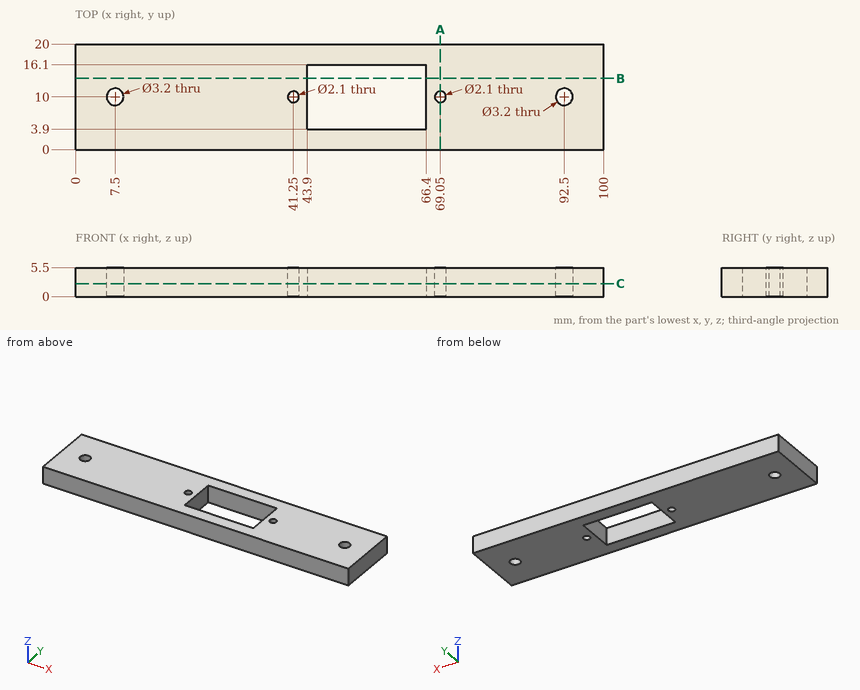
Input: dimensioned drawing with shaded views. Units: mm. Origin: part minimum x, y, z. Round coordinates to 2 decimals unless told otherwise and drop trailing zeros. Order: outer loops, then holes, each group sorted by start corner. A loop starts at its lowest first (then second) coordinate and runs counter-clockwise, first axis right, second up. Notation, with made-up numbers: (-37.75, -34.5) - (-22.75, -34.5) arc R22 ccw to (-22.75, -15.5) - close; hole circle Ø10 at (-3, 35.25). An arc over 180 degrees is marked (long way). Answer as a JSON object with one key per item and string values. Group by question number.
(1) Pin query (flat end, axial travel): P1, Ø2.5, axis at x = 7.5, y = 10, coming from the +Z side. Return the tip coordinate at first contact, or that it passes through.
(2) Cut plane A-A (x = 69.05). Return loops of the section in (y, z).
(3) Material intervals for probe 1 along Y at (x, z) = (61, 1.2); probe 2 along Y at (x, z) = (41.25, 1.2); probe 3 along X at (y, z) = (13.25, 5.35), sorted ascending. Write a range as from..to.
(4) Cut plane B-B (y = 13.5). Return loops of the section in (x, z), then the cut area to 3 significant figures.
(5) Cut plane C-C (z = 2.5). Return loops of the section in (x, y).
Here are the results:
{
 "1": {"P1": "passes through"},
 "2": {"outline": "(0, 0) - (8.95, 0) - (8.95, 5.5) - (0, 5.5) - close; (11.05, 0) - (20, 0) - (20, 5.5) - (11.05, 5.5) - close"},
 "3": {"probe 1": "y = 0..3.9, 16.1..20", "probe 2": "y = 0..8.95, 11.05..20", "probe 3": "x = 0..43.9, 66.4..100"},
 "4": {"outline": "(0, 0) - (43.9, 0) - (43.9, 5.5) - (0, 5.5) - close; (66.4, 0) - (100, 0) - (100, 5.5) - (66.4, 5.5) - close", "area": "426 mm^2"},
 "5": {"outline": "(0, 0) - (100, 0) - (100, 20) - (0, 20) - close; hole circle Ø3.2 at (7.5, 10); hole circle Ø2.1 at (41.25, 10); hole (43.9, 3.9) - (66.4, 3.9) - (66.4, 16.1) - (43.9, 16.1) - close; hole circle Ø2.1 at (69.05, 10); hole circle Ø3.2 at (92.5, 10)"}
}
